Autodesk Inventor part; units mm, degrees
ref_plane "YZ Plane" through (0, 0, 0) normal (1, 0, 0) x (0, 1, 0)
ref_plane "XZ Plane" through (0, 0, 0) normal (0, 1, 0) x (-1, 0, 0)
ref_plane "XY Plane" through (0, 0, 0) normal (0, 0, 1) x (1, 0, 0)
sketch "Sketch1" plane through (0, 0, 0) normal (0, 0, 1) x (1, 0, 0)
  line L0 (13.4, 187.5) -> (13.4, -187.5)
  line L1 (0, 187.5) -> (13.4, 187.5)
  line L2 (0, 187.5) -> (0, -187.5)
  line L3 (13.4, -187.5) -> (0, -187.5)
  line L4 (-6.6, 187.5) -> (-6.6, -187.5)
  line L5 (-11.3, 187.5) -> (-6.6, 187.5)
  line L6 (-11.3, 187.5) -> (-11.3, -187.5)
  line L7 (-6.6, -187.5) -> (-11.3, -187.5)
  line L8 (24.7, 187.5) -> (24.7, -187.5)
  line L9 (20, 187.5) -> (24.7, 187.5)
  line L10 (20, 187.5) -> (20, -187.5)
  line L11 (24.7, -187.5) -> (20, -187.5)
  line L12 (0, -104.7717) -> (51.7, -104.7717)
  line L13 (51.7, -104.7717) -> (51.7, -82.7717)
  line L14 (51.7, -82.7717) -> (0, -82.7717)
  line L15 (0, -82.7717) -> (0, -104.7717)
  line L16 (38.7, -104.7717) -> (38.7, -82.7717) construction
  line L17 (51.7, -93.7717) -> (36.1959, -93.7717) construction
  circle A0 centre (38.7, -101.9917) radius 2
  circle A1 centre (38.7, -85.5517) radius 2
  line L18 (13.4, -93.8117) -> (20, -93.8117) construction
  circle A2 centre (16.7, -93.8117) radius 2.5
  line L19 (6.7, -104.7717) -> (6.7, -82.7717)
  point P0 (0, 0)
  point P1 (0, -82.7717)
  dimension "d0" = 22
  dimension "d3" = 4
  dimension "d4" = 4
  dimension "d5" = 16.44
  dimension "d6" = 14
  dimension "d7" = 5
  dimension "d8" = 27
extrude "Extrusion1" add sketch "Sketch1" along normal blind 3 contours L14 L10 L12 L0 | L0 L12 L19 L14 | L14 L8 L12 L10 | L14 L13 L12 L8
sketch "Sketch2" plane through (0, 0, 0) normal (0, 0, -1) x (-1, 0, 0)
  line L0 (-14.2, 187.5) -> (-14.2, -187.5)
  line L1 (-19.2, 187.5) -> (-19.2, -187.5)
  line L2 (-51.7, -82.7717) -> (-6.7, -82.7717)
  line L3 (-6.7, -104.7717) -> (-51.7, -104.7717)
  line L4 (-51.7, -82.7717) -> (-6.7, -82.7717)
  line L5 (-14.3, -82.7717) -> (-19.1, -82.7717)
  line L6 (-19.1, -82.7717) -> (-19.1, -104.7717)
  line L7 (-19.1, -104.7717) -> (-14.3, -104.7717)
  line L8 (-14.3, -104.7717) -> (-14.3, -82.7717)
  circle A0 centre (-16.7, -93.8117) radius 2.5
  line L9 (-19.1, -96.3117) -> (-14.3, -96.3117)
  line L10 (-14.3, -96.3117) -> (-14.3, -91.3117)
  line L11 (-14.3, -91.3117) -> (-19.1, -91.3117)
  line L12 (-19.1, -91.3117) -> (-19.1, -96.3117)
  line L13 (-19.1, -96.3117) -> (-14.3, -91.3117) construction
  line L14 (-14.3, -96.3117) -> (-19.1, -91.3117) construction
  point P0 (0, 0)
  dimension "d9" = 0.1
  dimension "d10" = 0.1
extrude "Extrusion2" add sketch "Sketch2" along normal blind 1 contours L8 L11 L6 L2 | L3 L6 L9 L8
sketch "Sketch3" plane through (0, 0, 0) normal (0, 0, -1) x (-1, 0, 0)
  line L0 (-51.7, -104.7717) -> (-51.7, -82.7717)
  line L1 (-6.7, -104.7717) -> (-51.7, -104.7717)
  line L2 (-51.7, -82.7717) -> (-33.7, -82.7717)
  line L3 (-33.7, -82.7717) -> (-33.7, -104.7717)
  line L4 (-33.7, -104.7717) -> (-51.7, -104.7717)
  line L5 (-51.7, -104.7717) -> (-51.7, -82.7717)
  point P0 (0, 0)
  dimension "d13" = 18
extrude "Extrusion3" add sketch "Sketch3" along normal blind 6
thicken "Thicken1" operation cut thickness 6 both sides no extend neighbours no toward (0, 0, -1) faces at (38.1097, -101.6818, 0)
thicken "Thicken2" operation cut thickness 6 both sides no extend neighbours no toward (0, 0, -1) faces at (38.1097, -85.2418, 0)
chamfer "Chamfer1" distance 0.5 angle 45 6 edges at (33.7, -104.7717, -3) (33.7, -82.7717, -3) (51.7, -104.7717, -1.5) (51.7, -82.7717, -1.5) (6.7, -104.7717, 1.5) (6.7, -82.7717, 1.5)
properties part number "halter_induktivsensor_klein"
The model under review builds one solid part; all positions refer to its coordinate system, in mm. A direction names the side the tool comes from. Round coordinates to 2 decimals unless told otherwise and drop trailing zeros. Loops run counter-clockwise (first coordinate to the right, second up) from the corner with the lowest first, then second, coordinate; pieces in that order, holes last. Notation, with made-up numbers: M -10,-28 L 16,-28 A18 cw 16,-7 Z; hole C 88,24.25 d10. An arc over 180 degrees is marked long. Put each result on its own line as item: value.
Q1. Consider section C-C, the plane z = 1.5. Give the boundary of the cut face in (x, y), then the cut area to 3 significant figures.
Result set:
outline: M 6.7,-104.27 L 7.2,-104.77 L 51.2,-104.77 L 51.7,-104.27 L 51.7,-83.27 L 51.2,-82.77 L 7.2,-82.77 L 6.7,-83.27 Z; hole C 16.7,-93.81 d5; hole C 38.7,-101.99 d4; hole C 38.7,-85.55 d4
area: 945 mm²
Q2. Consider section D-D, the plane z = -2.5. Give the boundary of the cut face in (x, y), then the cut area to 3 significant figures.
Result set:
outline: M 33.7,-104.27 L 34.2,-104.77 L 51.2,-104.77 L 51.7,-104.27 L 51.7,-83.27 L 51.2,-82.77 L 34.2,-82.77 L 33.7,-83.27 Z; hole C 38.7,-101.99 d4; hole C 38.7,-85.55 d4
area: 370 mm²
Q3. Consider section B-B, the plane y = -86.75. Give the boundary of the cut face in (x, z).
Result set:
outline: M 6.7,0 L 14.3,0 L 14.3,-1 L 19.1,-1 L 19.1,0 L 33.7,0 L 33.7,-6 L 37.1,-6 L 37.1,3 L 6.7,3 Z; M 40.3,-6 L 51.7,-6 L 51.7,3 L 40.3,3 Z
Q4. Consider section A-A, the plane x = 38.7. Give the boundary of the cut face in (y, z), then the cut area to 3 significant figures.
Result set:
outline: M -104.77,-6 L -103.99,-6 L -103.99,3 L -104.77,3 Z; M -99.99,-6 L -87.55,-6 L -87.55,3 L -99.99,3 Z; M -83.55,-6 L -82.77,-6 L -82.77,3 L -83.55,3 Z
area: 126 mm²
Q5. Mouldability with a two-part tool opening along Y and no side actions: class faces 6 (the flat face through (51.7, -94, -1)), 7 (the cylindrical face through (38.44, -83.57, -1.44)), 8 (the flat face through (16.7, -91.312, -0.5)), 9 (the flat face through (34, -104.772, 1)) as released by +Y, released by -Y, zero draft, split by the parting line, or undercut.
Result set:
face 6: zero draft
face 7: undercut
face 8: undercut
face 9: released by -Y
Q6. Machinability: for faces 1 (the flat face through (16.7, -96.312, -0.5)), 2 (the flat face through (19.1, -87, -0.5)), 3 (the flat face through (29, -94, 3)), 4 (the cylindrical face through (38.266, -103.944, -1.437)), 5 (the flat face through (17, -87, -1)), which of the approach directions +Z, -Z, +X, -X, +Y, -Y give a long, thin tool a straight path to every point of the face, cutting with its end or side? Answer none if there is none.
Result set:
face 1: -Z, -X
face 2: -Z, +Y, -Y
face 3: +Z, +X, -X, +Y, -Y
face 4: +Z, -Z
face 5: -Z, -X, +Y, -Y
Q7. For pin 1 (2.5 mm diameter, centred on x = 38.7, y = -85.55, fed in from -Z); pin 2 (5 mm diameter, centred on y = -96.5, z = -4, fed in from -X); pin 3 (3 mm diameter, centred on x = 30.5, y = -88.5, fed in from -Z); pin 4 (2.5 mm diameter, centred on x = 17, y = -99.5, fed in from -Z), all flat-tipped, find the tip position at first contact; note any pin that passes through.
Result set:
pin 1: passes through
pin 2: stops at x = 33.7
pin 3: stops at z = 0
pin 4: stops at z = -1
Q8. To check wall thickness, follow L1, parallel to Y at x = 38.7, z = -2; L2, parallel to Y at x = 40, z = -5.5; L3, parallel to Y at x = 16.7, z = 1.25. State the ranges of each line that lie inside material, in increasing order.
Result set:
L1: y = -104.77 to -103.99, -99.99 to -87.55, -83.55 to -82.77
L2: y = -104.77 to -103.51, -100.47 to -87.07, -84.03 to -82.77
L3: y = -104.77 to -96.31, -91.31 to -82.77
